Can you work these out from the drawing? Everything is in mm from the part's minimum corner. A direction names the side the tool comes from. Coordinates: 2 decimals unless noted, no trailing zeros. Order: outer loops, then holes, each group sorted by start corner. A loop starts at its lowest first (then second) coordinate and runs counter-clockwise, first axis right, second up. Notation, with made-up numbers: (22, 26.5) -> (48, 26.5) arc R31 ccw to (48, 52.5) -> close; hole circle Ø7 at (49, 3). An arc over 180 degrees is marked (long way). Answer in a Markdown table with one row per item.
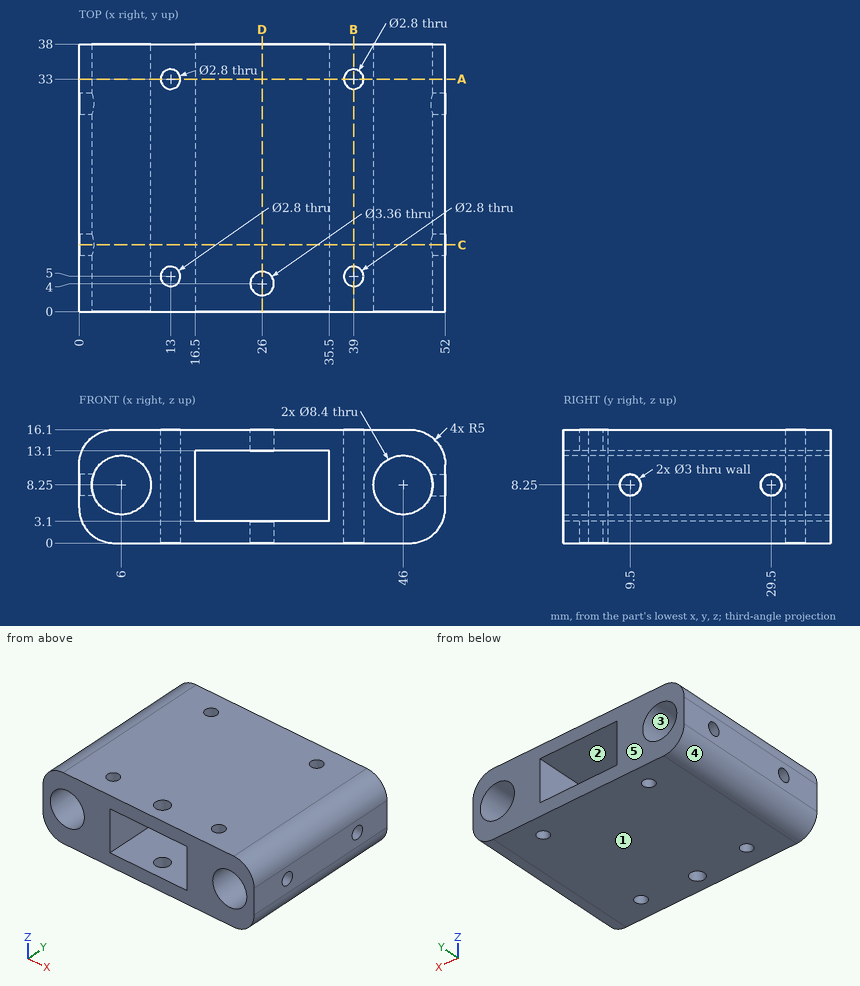
(1) Suppose I cut it at A-A (y = 33). Please give me the cut outline in (x, z).
Response values:
| item | result |
|---|---|
| outline | (0, 5) arc R5 ccw to (5, 0) -> (11.6, 0) -> (11.6, 16.1) -> (5, 16.1) arc R5 ccw to (0, 11.1) -> close; (14.4, 0) -> (37.6, 0) -> (37.6, 16.1) -> (14.4, 16.1) -> close; (40.4, 0) -> (47, 0) arc R5 ccw to (52, 5) -> (52, 11.1) arc R5 ccw to (47, 16.1) -> (40.4, 16.1) -> close; hole circle Ø8.4 at (6, 8.25); hole (16.5, 3.1) -> (35.5, 3.1) -> (35.5, 13.1) -> (16.5, 13.1) -> close; hole circle Ø8.4 at (46, 8.25) |
(2) Will these pins go through, and if not, where does the flat tip stop? pin 1 Ø1.8 at (y, z) = (9.5, 8.25) entering from -X; pin 2 Ø2.5 at (y, z) = (9.5, 8.25) entering from -X; pin 3 Ø1 at (x, z) = (33.5, 10) entering from -Y.
Response values:
| item | result |
|---|---|
| pin 1 | x = 10.1 |
| pin 2 | x = 10.01 |
| pin 3 | through |
(3) Suppose I cut it at D-D (x = 26). Please give me the cut outline in (y, z), and give its area (3 significant figures).
Response values:
| item | result |
|---|---|
| outline | (0, 0) -> (2.32, 0) -> (2.32, 3.1) -> (0, 3.1) -> close; (0, 13.1) -> (2.32, 13.1) -> (2.32, 16.1) -> (0, 16.1) -> close; (5.68, 0) -> (38, 0) -> (38, 3.1) -> (5.68, 3.1) -> close; (5.68, 13.1) -> (38, 13.1) -> (38, 16.1) -> (5.68, 16.1) -> close |
| area | 211 mm2 |
(4) We'd pull the mould along Z, two halves only. Please class the marked faces 3, 4 and 5: +Z half, -Z half, draft (parallel to the pull), parting line (faces both ways), or undercut.
Response values:
| item | result |
|---|---|
| face 3 | undercut |
| face 4 | -Z half |
| face 5 | draft |
(5) On a 3-axis mill with a long thin cutter (end or side, diameter ignored), from which of +Z, -Z, +X, -X, +Y, -Y can I reach the whole of each face in a straight line? I mean the marked faces 1 and 2. Say none if no direction works.
Response values:
| item | result |
|---|---|
| face 1 | -Z, +X, -X, +Y, -Y |
| face 2 | +Y, -Y |
(6) Suppose I cut it at B-B (x = 39). Please give me the cut outline in (y, z).
Response values:
| item | result |
|---|---|
| outline | (0, 0) -> (3.6, 0) -> (3.6, 16.1) -> (0, 16.1) -> close; (6.4, 0) -> (31.6, 0) -> (31.6, 16.1) -> (6.4, 16.1) -> close; (34.4, 0) -> (38, 0) -> (38, 16.1) -> (34.4, 16.1) -> close |
(7) Suppose I cut it at C-C (y = 9.5). Please give me the cut outline in (x, z).
Response values:
| item | result |
|---|---|
| outline | (0, 5) arc R5 ccw to (5, 0) -> (47, 0) arc R5 ccw to (52, 5) -> (52, 6.75) -> (49.92, 6.75) arc R4.2 cw (long way) to (49.92, 9.75) -> (52, 9.75) -> (52, 11.1) arc R5 ccw to (47, 16.1) -> (5, 16.1) arc R5 ccw to (0, 11.1) -> (0, 9.75) -> (2.08, 9.75) arc R4.2 cw (long way) to (2.08, 6.75) -> (0, 6.75) -> close; hole (16.5, 3.1) -> (35.5, 3.1) -> (35.5, 13.1) -> (16.5, 13.1) -> close |
(8) I need wall thicknesses on line 1 (Y direction, x = 13, z = 8.25); line 2 (Y direction, x = 51.5, z = 8.25); line 3 (Z direction, x = 27, y = 23). Which ranges of each line are inside material? Lowest first, please. Write a range as [from, to].
Response values:
| item | result |
|---|---|
| line 1 | [0, 3.6], [6.4, 31.6], [34.4, 38] |
| line 2 | [0, 8], [11, 28], [31, 38] |
| line 3 | [0, 3.1], [13.1, 16.1] |
